Verification items for the finished model (mm, model axes). Face numbers are marked on the shaded views. Coordinates: 2 decimals unless noted, no trailing zeros. Order: outer loops, then holes, each group sorted by start corner. A loop starts at its lowest first (then second) coordinate and runs counter-clockwise, first axis right, second up. Notation, with made-up numbers: M 33.25,84 L 91.25,84 A23 ccw 91.25,92 Z; hole C 68,-9.75 d3. An arc over 180 degrees is marked long. Write item = value, one per line.
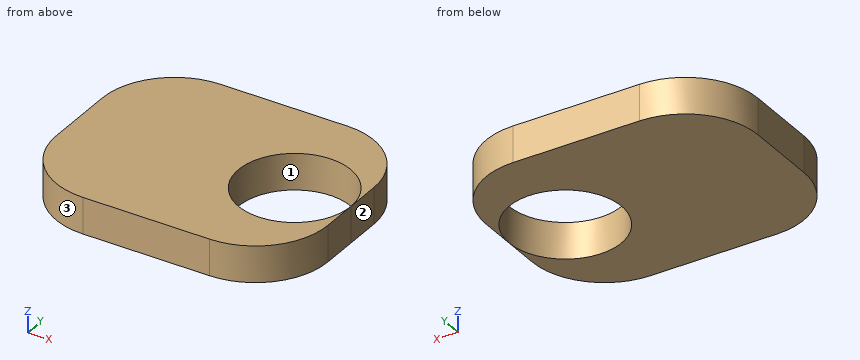
```python
from build123d import *

# Parameters (mm, degrees)
SKETCH_W  = 7.5
SKETCH_H  = 6
SKETCH_R  = 1.55
PAD_DEPTH = 1
FILLET_R  = 2


with BuildPart() as part:
    # Sketch → Pad (new body)
    with BuildSketch(Plane.XY):
        Rectangle(SKETCH_W, SKETCH_H)
        with Locations((2.2, 0)):
            Circle(SKETCH_R, mode=Mode.SUBTRACT)
    extrude(amount=PAD_DEPTH)

    # Fillet
    fillet_edges = [part.edges().sort_by_distance(p)[0] for p in [
        (-3.75, -3, 0.5),
        (3.75, -3, 0.5),
        (3.75, 3, 0.5),
        (-3.75, 3, 0.5),
    ]]
    fillet(fillet_edges, radius=FILLET_R)


solid = part.part
```
Item 1: Release check for a two-part mould opening along X. For the marked faces 1, 2 and 3 record: pulls with the +X half, pulls with the -X half, needs draft (parallel to the pull), parting line crosses it, or undercut.
Report:
face_1 = undercut
face_2 = pulls with the +X half
face_3 = pulls with the -X half
Item 2: Scan lines: L1, parallel to X at y = -1, z = 0.2; L2, parallel to Y at x = 2.2, z = 0.5; L3, parallel to Y at x = 3.25, z = 0.9. Record each from-to range of solid material in increasing order. Write a range as from..to.
Report:
L1 = -3.75..1.02, 3.38..3.75
L2 = -2.95..-1.55, 1.55..2.95
L3 = -2.32..-1.14, 1.14..2.32
Item 3: Sectioned sample at C-C, the plane x = 2.2. Enter the section's corners in (y, z), then the cut area to 3 significant figures.
Report:
outline = M -2.95,0 L -1.55,0 L -1.55,1 L -2.95,1 Z; M 1.55,0 L 2.95,0 L 2.95,1 L 1.55,1 Z
area = 2.80 mm^2
Item 4: Gauge pin test, flat end, axial feed: pin 1 (2 mm diameter, centred on x = 3, y = -1.5, fed in from -Z). Record the tip position at first contact, or that the pin passes through.
Report:
pin_1 = 0
Item 5: Sectioned sample at D-D, the plane y = -2. Enter the section's corners in (x, z).
Report:
outline = M -3.48,0 L 3.48,0 L 3.48,1 L -3.48,1 Z
